Design review of the part built by this model. Coordinates are the model's own, in mm. A direction names the side the tool comes from. Coordinates: 2 decimals unless noted, no trailing zeros. Order: outer loops, then holes, each group sorted by start corner. A loop starts at its lowest first (then second) coordinate and runs counter-clockwise, first axis right, second up. Notation, with made-up numbers: M 81.25,-13 L 93.25,-13 A21 ccw 93.25,4 Z; hole C 17,-0.75 d2. An arc over 180 degrees is marked long. Answer as a JSON object with one key per item and string values.
from build123d import *

# Parameters (mm, degrees)
SKETCH2_W               = 170
SKETCH2_H               = 170
SKETCH2_R               = 1.5
BOSS_EXTRUDE1_DEPTH     = 1.5
SKETCH5_R               = 15
CUT_EXTRUDE1_DEPTH      = 5
CUT_EXTRUDE1_DEPTH_BACK = 5
SKETCH6_R               = 1.5
CUT_EXTRUDE2_DEPTH      = 5
CUT_EXTRUDE2_DEPTH_BACK = 5
SKETCH7_R               = 1.5
CUT_EXTRUDE3_DEPTH      = 5
CUT_EXTRUDE3_DEPTH_BACK = 5
SKETCH8_R               = 1.5
CUT_EXTRUDE4_DEPTH      = 10
CUT_EXTRUDE4_DEPTH_BACK = 10
SKETCH9_W               = 170
SKETCH9_H               = 41.5
BOSS_EXTRUDE2_DEPTH     = 1.5
FILLET2_R               = 1
FILLET3_R               = 1
SKETCH10_W              = 170
SKETCH10_H              = 41.5
BOSS_EXTRUDE3_DEPTH     = 1.5
FILLET4_R               = 1
FILLET5_R               = 1
SKETCH15_R              = 1.5
CUT_EXTRUDE6_DEPTH      = 10000
CUT_EXTRUDE6_DEPTH_BACK = 10000


with BuildPart() as part:
    # Sketch2 → Boss-Extrude1 (new body)
    with BuildSketch(Plane(origin=(0, 0, 0), x_dir=(1, 0, 0), z_dir=(0, 1, 0))):
        with Locations((85, 85)):
            Rectangle(SKETCH2_W, SKETCH2_H)
        with Locations((63, 85)):
            Circle(SKETCH2_R, mode=Mode.SUBTRACT)
        with Locations((85, 63)):
            Circle(SKETCH2_R, mode=Mode.SUBTRACT)
        with Locations((85, 107)):
            Circle(SKETCH2_R, mode=Mode.SUBTRACT)
        with Locations((107, 85)):
            Circle(SKETCH2_R, mode=Mode.SUBTRACT)
    extrude(amount=BOSS_EXTRUDE1_DEPTH)

    # Sketch5 → Cut-Extrude1 (cut, two sides)
    with BuildSketch(Plane(origin=(0, 1.5, 0), x_dir=(1, 0, 0), z_dir=(0, 1, 0))) as cut_extrude1_sk:
        with Locations((85, 85)):
            Circle(SKETCH5_R)
    extrude(amount=CUT_EXTRUDE1_DEPTH, mode=Mode.SUBTRACT)
    extrude(cut_extrude1_sk.sketch, amount=-CUT_EXTRUDE1_DEPTH_BACK, mode=Mode.SUBTRACT)

    # Sketch6 → Cut-Extrude2 (cut, two sides)
    with BuildSketch(Plane(origin=(0, 1.5, 0), x_dir=(1, 0, 0), z_dir=(0, 1, 0))) as cut_extrude2_sk:
        with Locations((65, 94)):
            Circle(SKETCH6_R)
        with Locations((65, 76)):
            Circle(SKETCH6_R)
        with Locations((105, 76)):
            Circle(SKETCH6_R)
        with Locations((105, 94)):
            Circle(SKETCH6_R)
    extrude(amount=CUT_EXTRUDE2_DEPTH, mode=Mode.SUBTRACT)
    extrude(cut_extrude2_sk.sketch, amount=-CUT_EXTRUDE2_DEPTH_BACK, mode=Mode.SUBTRACT)

    # Sketch7 → Cut-Extrude3 (cut, two sides)
    with BuildSketch(Plane(origin=(0, 1.5, 0), x_dir=(1, 0, 0), z_dir=(0, 1, 0))) as cut_extrude3_sk:
        with Locations((6.5, 163.5)):
            Circle(SKETCH7_R)
        with Locations((163.5, 163.5)):
            Circle(SKETCH7_R)
        with Locations((163.5, 6.5)):
            Circle(SKETCH7_R)
        with Locations((6.5, 6.5)):
            Circle(SKETCH7_R)
    extrude(amount=CUT_EXTRUDE3_DEPTH, mode=Mode.SUBTRACT)
    extrude(cut_extrude3_sk.sketch, amount=-CUT_EXTRUDE3_DEPTH_BACK, mode=Mode.SUBTRACT)

    # Sketch8 → Cut-Extrude4 (cut, two sides)
    with BuildSketch(Plane(origin=(0, 1.5, 0), x_dir=(1, 0, 0), z_dir=(0, 1, 0))) as cut_extrude4_sk:
        with Locations((163.5, 18)):
            Circle(SKETCH8_R)
        with Locations((163.5, 152)):
            Circle(SKETCH8_R)
        with Locations((6.5, 152)):
            Circle(SKETCH8_R)
        with Locations((6.5, 18)):
            Circle(SKETCH8_R)
    extrude(amount=CUT_EXTRUDE4_DEPTH, mode=Mode.SUBTRACT)
    extrude(cut_extrude4_sk.sketch, amount=-CUT_EXTRUDE4_DEPTH_BACK, mode=Mode.SUBTRACT)

    # Sketch9 → Boss-Extrude2 (add)
    with BuildSketch(Plane(origin=(170, 0, 0), x_dir=(0, 0, -1), z_dir=(1, 0, 0))):
        with Locations((85, 20.75)):
            Rectangle(SKETCH9_W, SKETCH9_H)
    extrude(amount=BOSS_EXTRUDE2_DEPTH)

    # Fillet2
    fillet2_edges = [part.edges().sort_by_distance(p)[0] for p in [
        (170, 1.5, -85),
    ]]
    fillet(fillet2_edges, radius=FILLET2_R)

    # Fillet3
    fillet3_edges = [part.edges().sort_by_distance(p)[0] for p in [
        (171.5, 0, -85),
    ]]
    fillet(fillet3_edges, radius=FILLET3_R)

    # Sketch10 → Boss-Extrude3 (add)
    with BuildSketch(Plane.ZY):
        with Locations((-85, 20.75)):
            Rectangle(SKETCH10_W, SKETCH10_H)
    extrude(amount=BOSS_EXTRUDE3_DEPTH)

    # Fillet4
    fillet4_edges = [part.edges().sort_by_distance(p)[0] for p in [
        (0, 1.5, -85),
    ]]
    fillet(fillet4_edges, radius=FILLET4_R)

    # Fillet5
    fillet5_edges = [part.edges().sort_by_distance(p)[0] for p in [
        (-1.5, 0, -85),
    ]]
    fillet(fillet5_edges, radius=FILLET5_R)

    # Sketch15 → Cut-Extrude6 (cut, two sides)
    with BuildSketch(Plane.ZY.offset(1.5)) as cut_extrude6_sk:
        with Locations((-165, 16)):
            Circle(SKETCH15_R)
        with Locations((-165, 6)):
            Circle(SKETCH15_R)
        with Locations((-5, 16)):
            Circle(SKETCH15_R)
        with Locations((-5, 6)):
            Circle(SKETCH15_R)
    extrude(amount=CUT_EXTRUDE6_DEPTH, mode=Mode.SUBTRACT)
    extrude(cut_extrude6_sk.sketch, amount=-CUT_EXTRUDE6_DEPTH_BACK, mode=Mode.SUBTRACT)


solid = part.part
1) Tool access review of faces 4 (the flat face through (-1.5, 22, -86)), 5 (the flat face through (170, 22, -84)): name each direction out of +Z, -Z, +X, -X, +Y, -Y from which nothing blocks a thin tool from reaching the whole face with its end or side.
Taken from the geometry:
{"face 4": "+Z, -Z, -X, +Y, -Y", "face 5": "+Z, -Z, +Y"}
2) Add section A-A (y = 28). State the section outline as (x, z) points.
Taken from the geometry:
{"outline": "M -1.5,-170 L 0,-170 L 0,0 L -1.5,0 Z; M 170,-170 L 171.5,-170 L 171.5,0 L 170,0 Z"}
3) Mouldability with a two-part tool opening along Z and no side actions: class faces 1 (the flat face through (85, 1, 0)), 2 (the cylindrical face through (81.748, 0.76, -70.357)), 3 (the flat face through (65, 1.5, -86)) as released by +Z, released by -Z, zero draft, split by the parting line, or undercut.
Taken from the geometry:
{"face 1": "released by +Z", "face 2": "undercut", "face 3": "zero draft"}
4) Add section B-B (z = -22.5). State the section outline as (x, y) points.
Taken from the geometry:
{"outline": "M -1.5,1 A1 ccw -0.5,0 L 170.5,0 A1 ccw 171.5,1 L 171.5,41.5 L 170,41.5 L 170,2.5 A1 cw 169,1.5 L 1,1.5 A1 cw 0,2.5 L 0,41.5 L -1.5,41.5 Z"}
5) Add section C-C (x = 20.5). State the section outline as (y, z) points.
Taken from the geometry:
{"outline": "M 0,-170 L 1.5,-170 L 1.5,0 L 0,0 Z"}
6) To check wall thickness, follow L1, parallel to Z at x = 85, y = 0.75; L2, parallel to Z at x = 6.5, y = 0.85; L3, parallel to X at y = 21, z = -144.5. State the ranges of each line that lie inside material, in increasing order.
Taken from the geometry:
{"L1": "z = -170 to -108.5, -105.5 to -100, -70 to -64.5, -61.5 to 0", "L2": "z = -170 to -165, -162 to -153.5, -150.5 to -19.5, -16.5 to -8, -5 to 0", "L3": "x = -1.5 to 0, 170 to 171.5"}
7) Insertion check: pin 1 Ø5 at (x, z) = (63, -85) entering from +Y. The pin has a flat end and moves straight along its axis. Give the tip position at first contact, or say it passes through.
Taken from the geometry:
{"pin 1": "stops at y = 1.5"}
